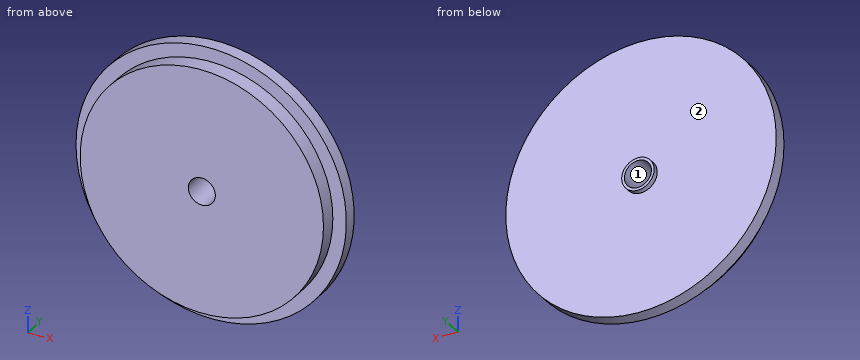
Autodesk Inventor part; units mm, degrees
ref_plane "YZ Plane" through (0, 0, 0) normal (1, 0, 0) x (0, 1, 0)
ref_plane "XZ Plane" through (0, 0, 0) normal (0, 1, 0) x (-1, 0, 0)
ref_plane "XY Plane" through (0, 0, 0) normal (0, 0, 1) x (1, 0, 0)
sketch "Boceto1" plane through (0, 0, 0) normal (0, 1, 0) x (-1, 0, 0)
  line L0 (0, 0) -> (100, 0) construction
  line L1 (100, 0) -> (100, -100) construction
  line L2 (100, -100) -> (0, -100) construction
  line L3 (0, -100) -> (0, 0) construction
  line L4 (100, -100) -> (0, 0) construction
  line L5 (100, 0) -> (0, -100) construction
  circle A0 centre (50, -50) radius 50
  dimension "d0" = 100
  dimension "d1" = 100
  dimension "d2" = 100
extrude "Extrusión1" add sketch "Boceto1" along normal blind 5
sketch "Boceto2" plane through (-50, 0, -50) normal (0, -1, 0) x (1, 0, 0)
  circle A0 centre (0, 0) radius 45
  point P0 (50, 50)
  dimension "d5" = 90
extrude "Extrusión2" add sketch "Boceto2" along normal blind 6
thread "Rosca1"
sketch "Boceto3" plane through (-50, 5, -50) normal (0, 1, 0) x (1, 0, 0)
  circle A0 centre (0, 0) radius 6
  point P0 (50, -50)
  dimension "d10" = 12
extrude "Extrusión3" add sketch "Boceto3" along normal blind 2
sketch "Boceto4" plane through (-50, 7, -50) normal (0, 1, 0) x (1, 0, 0)
  circle A0 centre (0, 0) radius 5
  point P0 (50, -50)
  dimension "d13" = 10
extrude "Extrusión4" cut sketch "Boceto4" against normal through all
thread "Rosca2"
CAD build for the part. Positions are in the model's coordinates, mm. Face numbers are marked on the shaded views. Coordinates: 2 decimals unless noted, no trailing zeros. Loops run counter-clockwise (first coordinate to the right, second up) from the corner with the lowest first, then second, coordinate; pieces in that order, holes last. Notation, with made-up numbers: (-23, 0) -> (-3, 0) arc R29 cw to (-3, 25) -> close; hole circle Ø3 at (-3.75, 37.5). An arc over 180 degrees is marked (long way). One line per item, written item: value.
1. Slice it at B-B on x = -50. Write the cut outline in (y, z), and give its area (3 significant figures).
Answers:
outline: (-6, -95) -> (0, -95) -> (0, -100) -> (5, -100) -> (5, -56) -> (7, -56) -> (7, -55) -> (-6, -55) -> close; (-6, -45) -> (7, -45) -> (7, -44) -> (5, -44) -> (5, 0) -> (0, 0) -> (0, -5) -> (-6, -5) -> close
area: 934 mm^2
2. Slice it at A-A on z = -50. Write the cut outline in (x, y), and give its area (3 significant figures).
Answers:
outline: (-100, 0) -> (-95, 0) -> (-95, -6) -> (-55, -6) -> (-55, 7) -> (-56, 7) -> (-56, 5) -> (-100, 5) -> close; (-45, -6) -> (-5, -6) -> (-5, 0) -> (0, 0) -> (0, 5) -> (-44, 5) -> (-44, 7) -> (-45, 7) -> close
area: 934 mm^2
3. Pull direction X, two halves, no side cores. Call the marked faces 1 and 2: pulls with the +X half, pulls with the -X half, needs draft (parallel to the pull), parting line crosses it, or undercut.
Answers:
face 1: undercut
face 2: needs draft
4. Slice it at C-C on y = -3.25. Write the cut outline in (x, z).
Answers:
outline: circle Ø90 at (-50, -50); hole circle Ø10 at (-50, -50)
5. Drill centre lines: line 1 (Z direction, x = -50.5, y = 2); line 2 (Y direction, x = -56, z = -78.5); line 3 (Y direction, x = -66.5, z = -5). Where is each one in solid material? Low to high. Write a range as [from, to].
Answers:
line 1: z = [-100, -54.97], [-45.03, 0]
line 2: y = [-6, 5]
line 3: y = [0, 5]
6. Slice it at D-D on z = -9.5. Write the cut outline in (x, y), and give its area (3 significant figures).
Answers:
outline: (-79.32, 0) -> (-69.62, 0) -> (-69.62, -6) -> (-30.38, -6) -> (-30.38, 0) -> (-20.68, 0) -> (-20.68, 5) -> (-79.32, 5) -> close
area: 529 mm^2
7. Flat gauge pins, fed straight in: P1, Ø16, axis at x = -50, z = -50, coming from the -Y side; P2, Ø1, axis at y = -4, z = -80, coming from the +X side; P3, Ø2, axis at y = 5.5, z = -32.5, coming from the +X side; P4, Ø3, axis at x = -38.5, z = -25.5, coming from the +Y side. Where does each tip first touch, or does it go through?
Answers:
P1: stops at y = -6
P2: stops at x = -16.02
P3: stops at x = -2.85
P4: stops at y = 5
